```python
from build123d import *

# Parameters (mm, degrees)
SKETCH_1_W          = 22
SKETCH_1_H          = 53
SKETCH_1_R          = 2.5
SKETCH_1_R_2        = 5.5
SKETCH_1_R_3        = 1.5
EXTRUDE_1_DEPTH     = 8
CUT_EXTRUDE_START   = -10
CUT_EXTRUDE_1_DEPTH = 10


with BuildPart() as part:
    # 草图1 → 凸台-拉伸1 (new body)
    with BuildSketch(Plane.XY):
        with Locations((-7.008849558, -2.699115044)):
            Rectangle(SKETCH_1_W, SKETCH_1_H)
        with Locations((-12.508849558, -19.199115044)):
            Circle(SKETCH_1_R, mode=Mode.SUBTRACT)
        with Locations((-1.508849558, -19.199115044)):
            Circle(SKETCH_1_R, mode=Mode.SUBTRACT)
        with Locations((-7.008849558, 12.800884956)):
            Circle(SKETCH_1_R_2, mode=Mode.SUBTRACT)
        with Locations((-7.008849558, 20.858941567)):
            Circle(SKETCH_1_R_3, mode=Mode.SUBTRACT)
        with Locations((1.049207054, 12.800884956)):
            Circle(SKETCH_1_R_3, mode=Mode.SUBTRACT)
        with Locations((-7.008849558, 4.742828344)):
            Circle(SKETCH_1_R_3, mode=Mode.SUBTRACT)
        with Locations((-15.066906169, 12.800884956)):
            Circle(SKETCH_1_R_3, mode=Mode.SUBTRACT)
    extrude(amount=EXTRUDE_1_DEPTH)

    # 草图2 → 切除-拉伸1 (cut)
    with BuildSketch(Plane.XY.offset(8).offset(CUT_EXTRUDE_START)):
        with BuildLine():
            Line((-12.508849558, 12.800884956), (-12.508849558, 23.800884956))
            Line((-12.508849558, 23.800884956), (-1.508849558, 23.800884956))
            Line((-1.508849558, 23.800884956), (-1.508849558, 12.800884956))
            ThreePointArc((-1.508849558, 12.800884956), (-7.008849558, 7.300884956), (-12.508849558, 12.800884956))
        make_face()
    extrude(amount=CUT_EXTRUDE_1_DEPTH, mode=Mode.SUBTRACT)


solid = part.part
```
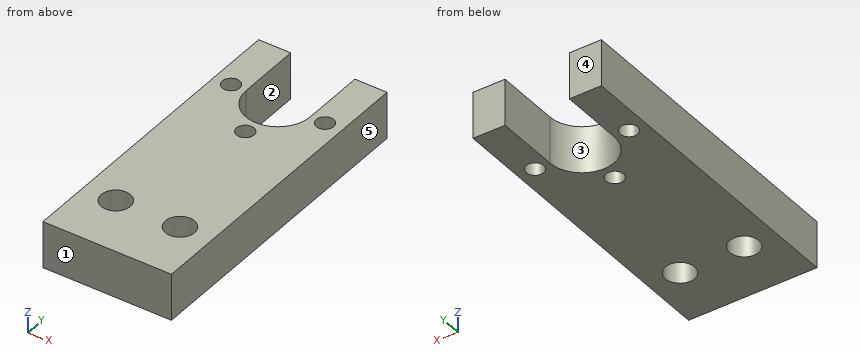
Input: part model. Units: mm. Frame: model coordinates. Face numbers are marked on the shaded views. A direction names the side the tool comes from. Coordinates: 2 decimals unless noted, no trailing zeros. Write each loop counter-clockwise with the first axis right and the second up, starting at its lowest first coordinate (ties: lowest second). Pieces come first, ordered by that corner, then holes. Notation, with made-up numbers: (4, 85) -> (54, 85) arc R33 ccw to (54, 113) -> close; hole circle Ø1 at (86, 12). An arc over 180 degrees is marked (long way). Answer as a JSON object with one key per item and string values.
1. First-contact query: P1, Ø4, axis at x = -12.51, y = -19.2, coming from the +Z side. Flat tip, straight axial feed; report the tip coordinate or a pass-through.
Result set:
{"P1": "passes through"}
2. Section A-A on z = 3.5. Return the cut outline in (x, y).
Result set:
{"outline": "(-18.01, -29.2) -> (3.99, -29.2) -> (3.99, 23.8) -> (-1.51, 23.8) -> (-1.51, 12.8) arc R5.5 cw to (-12.51, 12.8) -> (-12.51, 23.8) -> (-18.01, 23.8) -> close; hole circle Ø3 at (-15.07, 12.8); hole circle Ø5 at (-12.51, -19.2); hole circle Ø3 at (-7.01, 4.74); hole circle Ø5 at (-1.51, -19.2); hole circle Ø3 at (1.05, 12.8)"}
3. Access query for the marked faces 1 and 2. Directions: +Z, -Z, +X, -X, +Y, -Y. A direction counts if a zero-diameter tool reaches every point of the face in a straight line with its end or side. Return the directions, or none.
Result set:
{"face 1": "+Z, -Z, +X, -X, -Y", "face 2": "+Z, -Z, +Y"}
4. Section C-C on x = 0.5. Return the cut outline in (y, z).
Result set:
{"outline": "(-29.2, 0) -> (-20.69, 0) -> (-20.69, 8) -> (-29.2, 8) -> close; (-17.71, 0) -> (11.41, 0) -> (11.41, 8) -> (-17.71, 8) -> close; (14.2, 0) -> (23.8, 0) -> (23.8, 8) -> (14.2, 8) -> close"}
5. Material intervals for line 1 (X direction, y = 13.5, z = 3.5); line 2 (Y direction, x = 0.25, z = 4.25); line 3 (Y direction, x = -7, z = 5), sorted ascending. Write a range as from..to.
Result set:
{"line 1": "x = -18.01..-16.39, -13.74..-12.51, -1.51..-0.28, 2.38..3.99", "line 2": "y = -29.2..-20.98, -17.42..11.53, 14.07..23.8", "line 3": "y = -29.2..3.24, 6.24..7.3"}
6. Mould query, pull axis X, two halves, no side actions, for the marked faces 3, 4 and 5. Classes: released by +X, released by -X, zero draft, split by the parting line, or undercut.
Result set:
{"face 3": "undercut", "face 4": "zero draft", "face 5": "released by +X"}
7. Section D-D on x = -3.25. Return the cut outline in (y, z).
Result set:
{"outline": "(-29.2, 0) -> (-20.99, 0) -> (-20.99, 8) -> (-29.2, 8) -> close; (-17.41, 0) -> (8.79, 0) -> (8.79, 8) -> (-17.41, 8) -> close"}
8. Section B-B on x = -6. Return the cut outline in (y, z), then the cut area to 3 significant figures.
Result set:
{"outline": "(-29.2, 0) -> (3.63, 0) -> (3.63, 8) -> (-29.2, 8) -> close; (5.85, 0) -> (7.39, 0) -> (7.39, 8) -> (5.85, 8) -> close", "area": "275 mm2"}
